```python
from build123d import *

# Parameters (mm, degrees)
SKETCH1_W           = 243.84
SKETCH1_H           = 243.84
BOSS_EXTRUDE1_DEPTH = 6.35
CUT_EXTRUDE1_REACH  = 346.9
SKETCH5_W           = 10.16
SKETCH5_H           = 10.16


with BuildPart() as part:
    # Sketch1 → Boss-Extrude1 (new body)
    with BuildSketch(Plane(origin=(0, 0, 0), x_dir=(1, 0, 0), z_dir=(0, 1, 0))):
        with Locations((121.92, 121.92)):
            Rectangle(SKETCH1_W, SKETCH1_H)
    extrude(amount=BOSS_EXTRUDE1_DEPTH)

    # Sketch5 → Cut-Extrude1 (cut, up to next)
    with BuildSketch(Plane(origin=(0, 6.35, 0), x_dir=(1, 0, 0), z_dir=(0, 1, 0)), mode=Mode.PRIVATE) as cut_extrude1_sk1:
        with Locations((6.35, 6.35)):
            Rectangle(SKETCH5_W, SKETCH5_H)
    cut_extrude1_tool1 = extrude(cut_extrude1_sk1.sketch, amount=-CUT_EXTRUDE1_REACH, mode=Mode.PRIVATE) & part.part
    # Sketch5 → Cut-Extrude1 (cut, up to next)
    with BuildSketch(Plane(origin=(0, 6.35, 0), x_dir=(1, 0, 0), z_dir=(0, 1, 0)), mode=Mode.PRIVATE) as cut_extrude1_sk2:
        with Locations((78.74, 6.35)):
            Rectangle(SKETCH5_W, SKETCH5_H)
    cut_extrude1_tool2 = extrude(cut_extrude1_sk2.sketch, amount=-CUT_EXTRUDE1_REACH, mode=Mode.PRIVATE) & part.part
    # Sketch5 → Cut-Extrude1 (cut, up to next)
    with BuildSketch(Plane(origin=(0, 6.35, 0), x_dir=(1, 0, 0), z_dir=(0, 1, 0)), mode=Mode.PRIVATE) as cut_extrude1_sk3:
        with Locations((210.82, 6.35)):
            Rectangle(SKETCH5_W, SKETCH5_H)
    cut_extrude1_tool3 = extrude(cut_extrude1_sk3.sketch, amount=-CUT_EXTRUDE1_REACH, mode=Mode.PRIVATE) & part.part
    # Sketch5 → Cut-Extrude1 (cut, up to next)
    with BuildSketch(Plane(origin=(0, 6.35, 0), x_dir=(1, 0, 0), z_dir=(0, 1, 0)), mode=Mode.PRIVATE) as cut_extrude1_sk4:
        with Locations((233.68, 163.83)):
            Rectangle(SKETCH5_W, SKETCH5_H)
    cut_extrude1_tool4 = extrude(cut_extrude1_sk4.sketch, amount=-CUT_EXTRUDE1_REACH, mode=Mode.PRIVATE) & part.part
    # Sketch5 → Cut-Extrude1 (cut, up to next)
    with BuildSketch(Plane(origin=(0, 6.35, 0), x_dir=(1, 0, 0), z_dir=(0, 1, 0)), mode=Mode.PRIVATE) as cut_extrude1_sk5:
        with Locations((233.68, 209.55)):
            Rectangle(SKETCH5_W, SKETCH5_H)
    cut_extrude1_tool5 = extrude(cut_extrude1_sk5.sketch, amount=-CUT_EXTRUDE1_REACH, mode=Mode.PRIVATE) & part.part
    # Sketch5 → Cut-Extrude1 (cut, up to next)
    with BuildSketch(Plane(origin=(0, 6.35, 0), x_dir=(1, 0, 0), z_dir=(0, 1, 0)), mode=Mode.PRIVATE) as cut_extrude1_sk6:
        with Locations((78.74, 209.55)):
            Rectangle(SKETCH5_W, SKETCH5_H)
    cut_extrude1_tool6 = extrude(cut_extrude1_sk6.sketch, amount=-CUT_EXTRUDE1_REACH, mode=Mode.PRIVATE) & part.part
    # Sketch5 → Cut-Extrude1 (cut, up to next)
    with BuildSketch(Plane(origin=(0, 6.35, 0), x_dir=(1, 0, 0), z_dir=(0, 1, 0)), mode=Mode.PRIVATE) as cut_extrude1_sk7:
        with Locations((78.74, 163.83)):
            Rectangle(SKETCH5_W, SKETCH5_H)
    cut_extrude1_tool7 = extrude(cut_extrude1_sk7.sketch, amount=-CUT_EXTRUDE1_REACH, mode=Mode.PRIVATE) & part.part
    # Sketch5 → Cut-Extrude1 (cut, up to next)
    with BuildSketch(Plane(origin=(0, 6.35, 0), x_dir=(1, 0, 0), z_dir=(0, 1, 0)), mode=Mode.PRIVATE) as cut_extrude1_sk8:
        with Locations((6.35, 163.83)):
            Rectangle(SKETCH5_W, SKETCH5_H)
    cut_extrude1_tool8 = extrude(cut_extrude1_sk8.sketch, amount=-CUT_EXTRUDE1_REACH, mode=Mode.PRIVATE) & part.part
    # Sketch5 → Cut-Extrude1 (cut, up to next)
    with BuildSketch(Plane(origin=(0, 6.35, 0), x_dir=(1, 0, 0), z_dir=(0, 1, 0)), mode=Mode.PRIVATE) as cut_extrude1_sk9:
        with Locations((78.74, 229.87)):
            Rectangle(SKETCH5_W, SKETCH5_H)
    cut_extrude1_tool9 = extrude(cut_extrude1_sk9.sketch, amount=-CUT_EXTRUDE1_REACH, mode=Mode.PRIVATE) & part.part
    add(cut_extrude1_tool1.solids().sort_by_distance((6.35, 6.35, -6.35))[0], mode=Mode.SUBTRACT)
    add(cut_extrude1_tool2.solids().sort_by_distance((78.74, 6.35, -6.35))[0], mode=Mode.SUBTRACT)
    add(cut_extrude1_tool3.solids().sort_by_distance((210.82, 6.35, -6.35))[0], mode=Mode.SUBTRACT)
    add(cut_extrude1_tool4.solids().sort_by_distance((233.68, 6.35, -163.83))[0], mode=Mode.SUBTRACT)
    add(cut_extrude1_tool5.solids().sort_by_distance((233.68, 6.35, -209.55))[0], mode=Mode.SUBTRACT)
    add(cut_extrude1_tool6.solids().sort_by_distance((78.74, 6.35, -209.55))[0], mode=Mode.SUBTRACT)
    add(cut_extrude1_tool7.solids().sort_by_distance((78.74, 6.35, -163.83))[0], mode=Mode.SUBTRACT)
    add(cut_extrude1_tool8.solids().sort_by_distance((6.35, 6.35, -163.83))[0], mode=Mode.SUBTRACT)
    add(cut_extrude1_tool9.solids().sort_by_distance((78.74, 6.35, -229.87))[0], mode=Mode.SUBTRACT)


solid = part.part
```
Verification items for the finished model (mm, model axes). Coordinates: 2 decimals unless noted, no trailing zeros. Answer in a Markdown table with one row per item. Add a question column.
1. Section check A-A, the plane y = 3.5. Give the number of separate pieces and of enclosed holes in the cut face, then the cut area to 3 significant figures.
2. Draft check along Z on faces 1 (the face through (205.74, 3, -6)), 2 (the face through (0, 3, -120)). Enter one of: +Z half, -Z half, draft (parallel to the pull), parting line (faces both ways), or undercut.
3. Material ranges on probe 1 along Z at (x, y) = (83, 1.5), recorded low to high. Write a range as [from, to].
Derived:
| question | item | result |
|---|---|---|
| 1 | separate pieces | 1 |
| 1 | enclosed holes | 9 |
| 1 | area | 58,500 mm² |
| 2 | face 1 | undercut |
| 2 | face 2 | draft |
| 3 | probe 1 | z = [-243.84, -234.95], [-224.79, -214.63], [-204.47, -168.91], [-158.75, -11.43], [-1.27, 0] |
